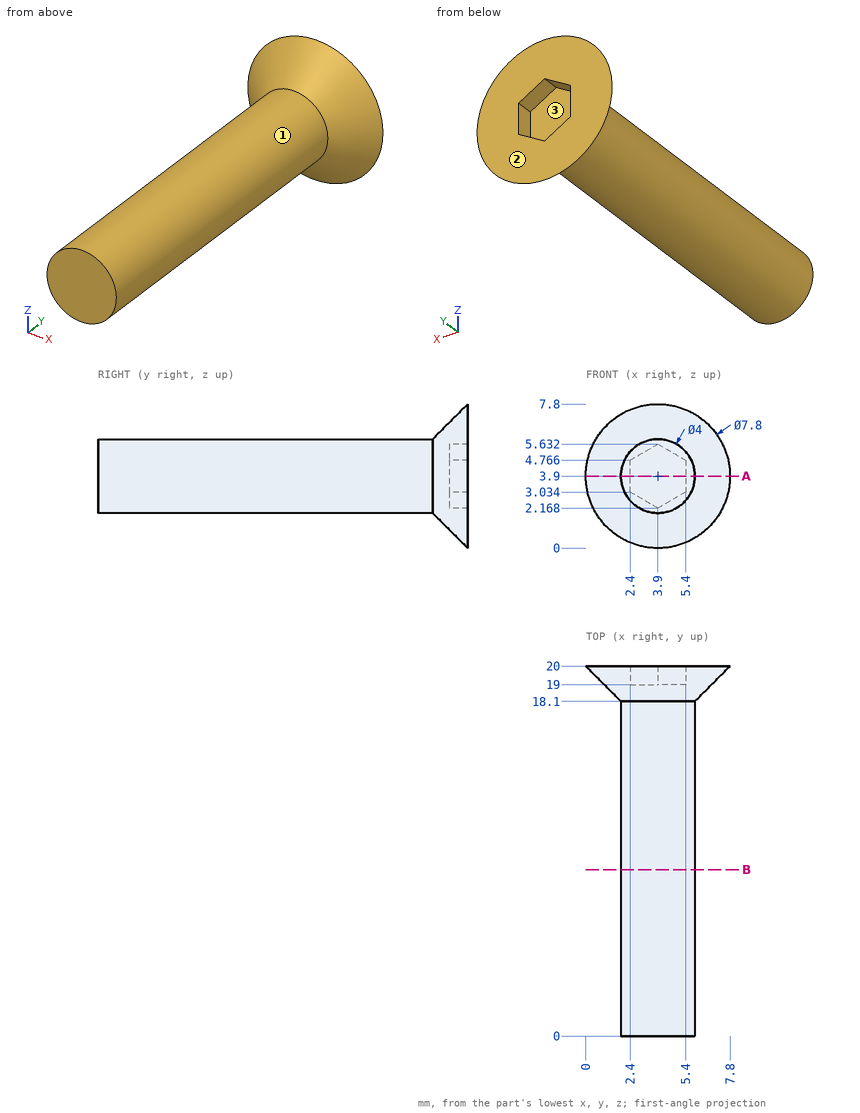
Geometry: see drawing. Coordinates: mm, zero at the bounding-box minimum. Coordinates: 2 decimals unless noted, no trailing zeros. Loops run counter-clockwise (first coordinate to the right, second up) from the corner with the lowest first, then second, coordinate; pieces in that order, holes last. Notation, with made-up numbers: M 88.5,9 L 146.5,9 A14 ccw 146.5,14 Z; hole C -14.5,82 d11. An arc over 180 degrees is marked long. Answer in a Markdown table with one row per item.
Q1. Draft query along Z for the marked faces 1, 2 and 3. Return one class per face: pulls with the +Z half, pulls with the -Z half, needs draft (parallel to the pull), parting line crosses it, or undercut.
Answers below:
| item | result |
|---|---|
| face 1 | parting line crosses it |
| face 2 | needs draft |
| face 3 | undercut |
Q2. Section A-A on z = 3.9. Return the cut outline in (x, y), plus the area to 3 significant figures.
Answers below:
| item | result |
|---|---|
| outline | M 0,20 L 1.9,18.1 L 1.9,0 L 5.9,0 L 5.9,18.1 L 7.8,20 L 5.4,20 L 5.4,19 L 2.4,19 L 2.4,20 Z |
| area | 80.6 mm^2 |
Q3. Ray query, probe 1 along Y at (x, z) = (3.25, 3.75); probe 2 along Y at (x, z) = (3.75, 1); probe 3 along Z at (x, y) = (4.5, 3.5). Return the intervals inside material, ascending. Write a range as from..to.
Answers below:
| item | result |
|---|---|
| probe 1 | y = 0..19 |
| probe 2 | y = 19..20 |
| probe 3 | z = 1.99..5.81 |
Q4. Section B-B on y = 9. Return the cut outline in (x, z), plus the area to 3 significant figures.
Answers below:
| item | result |
|---|---|
| outline | C 3.9,3.9 d4 |
| area | 12.6 mm^2 |
Q5. First-contact query: pin 1 (1.5 mm diameter, centred on y = 17.5, z = 4, fed in from -X); pin 2 (1.5 mm diameter, centred on x = 2, z = 6, fed in from -Y); pin 3 (3 mm diameter, centred on x = 6, y = 9.5, fed in from +Z). Flat tips, straight axial feed; report the tip coordinate or a pass-through.
Answers below:
| item | result |
|---|---|
| pin 1 | stops at x = 1.75 |
| pin 2 | stops at y = 18.18 |
| pin 3 | stops at z = 5.81 |
